from build123d import *

# Parameters (mm, degrees)
SKETCH_1_W          = 25
SKETCH_1_H          = 25
EXTRUDE_1_DEPTH     = 10
SKETCH_2_W          = 10
SKETCH_2_H          = 25
EXTRUDE_2_DEPTH     = 120
SKETCH_6_R          = 5.5
CUT_EXTRUDE_1_DEPTH = 121


with BuildPart() as part:
    # ｽｹｯﾁ1 → ﾎﾞｽ - 押し出し1 (new body)
    with BuildSketch(Plane.XY):
        with Locations((-26.305611861, 22.91927309)):
            Rectangle(SKETCH_1_W, SKETCH_1_H)
    extrude(amount=EXTRUDE_1_DEPTH)

    # ｽｹｯﾁ2 → ﾎﾞｽ - 押し出し2 (add)
    with BuildSketch(Plane(origin=(0, 0, 0), x_dir=(-1, 0, 0), z_dir=(0, 0, -1))):
        with Locations((43.805611861, 22.91927309)):
            Rectangle(SKETCH_2_W, SKETCH_2_H)
    extrude(amount=-EXTRUDE_2_DEPTH)

    # ｽｹｯﾁ6 → ｶｯﾄ - 押し出し1 (cut, through all)
    with BuildSketch(Plane(origin=(0, 0, 0), x_dir=(-1, 0, 0), z_dir=(0, 0, -1))):
        with Locations((26.305611861, 22.91927309)):
            Circle(SKETCH_6_R)
    extrude(amount=-CUT_EXTRUDE_1_DEPTH, mode=Mode.SUBTRACT)


solid = part.part
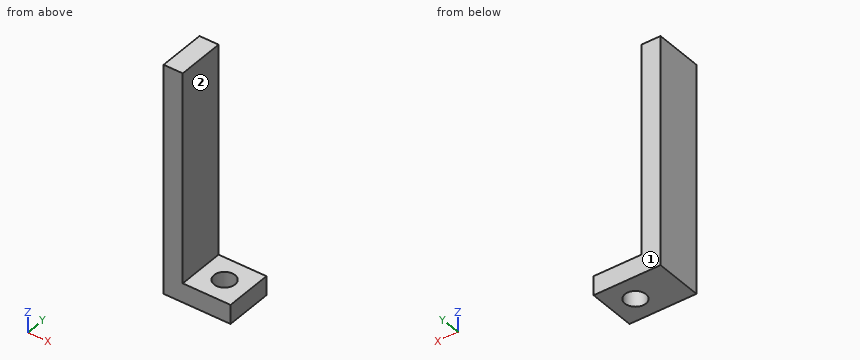
Design review of the part built by this model. Coordinates are the model's own, in mm. Face numbers are marked on the shaded views. A direction names the side the tool comes from. Give positions to 0.01 mm unless a question says otherwise; leave off trailing zeros. Order: outer loops, then holes, each group sorted by start corner. A loop starts at its lowest first (then second) coordinate and runs counter-clockwise, first axis right, second up. Notation, with made-up numbers: (27.5, 73) - (63.5, 73) arc R10 ccw to (63.5, 80) - close; hole circle Ø8 at (-9.75, -27.75). An arc over 180 degrees is marked (long way). Write item = value, one per line. Start each with the question number.
Q1. We need section B-B on x = -29. State the section outline as (y, z) points.
Q2. Tool access review of the marked faces 1 and 2: name each direction out of +Z, -Z, +X, -X, +Y, -Y from which nothing blocks a thin tool from reaching the whole face with its end or side.
Q3. To check wall thickness, follow L1, parallel to X at y = 11.5, z = 33.5; L2, parallel to Z at x = -17.5, y = 32; L3, parallel to Y at x = -23, z = 5. State the ranges of each line that lie inside material, in increasing order. Write a range as from..to.
Q4. We need section D-D on y = 26.25. State the section outline as (x, z) points, plus the area to 3 significant figures.
Q5. Clearance check with flat-ended pins moving along their axes: pin 1 Ø3 at (x, y) = (-24, 26.5) entering from +Z; pin 2 Ø7.5 at (y, z) = (23.5, 46.5) entering from +X. State where each tip first meets the part, or that it passes through.
Q6. We need section A-A on y = 20.75. State the section outline as (x, z) points.
Q7. We need section C-C on z = 89.5. State the section outline as (x, y) points.
Working result:
q1.outline = (10.42, 0) - (18.12, 0) - (18.12, 10) - (10.42, 10) - close; (27.71, 0) - (35.42, 0) - (35.42, 10) - (27.71, 10) - close
q2.face_1 = +Z, -Z, +X, -X, +Y
q2.face_2 = +Z, +X, +Y, -Y
q3.L1 = -48.81..-38.81
q3.L2 = 0..10
q3.L3 = 10.42..18.52, 27.32..35.42
q4.outline = (-48.81, 0) - (-30.68, 0) - (-30.68, 10) - (-38.81, 10) - (-38.81, 120) - (-48.81, 120) - close; (-21.93, 0) - (-13.81, 0) - (-13.81, 10) - (-21.93, 10) - close
q4.area = 1,360 mm²
q5.pin_1 = 10
q5.pin_2 = -38.81
q6.outline = (-48.81, 0) - (-31.36, 0) - (-31.36, 10) - (-38.81, 10) - (-38.81, 120) - (-48.81, 120) - close; (-21.25, 0) - (-13.81, 0) - (-13.81, 10) - (-21.25, 10) - close
q7.outline = (-48.81, 10.42) - (-38.81, 10.42) - (-38.81, 35.42) - (-48.81, 35.42) - close
